Verification items for the finished model (mm, model axes). Face numbers are marked on the shaded views. Coordinates: 2 decimals unless noted, no trailing zeros. Order: outer loops, then holes, each group sorted by start corner. A loop starts at its lowest first (then second) coordinate and runs counter-clockwise, first axis right, second up. Notation, with made-up numbers: M -14.75,60.5 L 37.25,60.5 A26 ccw 37.25,79.5 Z; hole C 48.5,17 d5. An arc over 180 degrees is marked long. Return JSON: item names as keys, results as strings. Group by question number.
1. Material ranges on line 1 along Z through (x, y) = (3, 14.75); line 2 along Z through (x, y) = (3.75, 12.5); line 3 along X through (y, z) = (6, -2), recorded low to high.
2. Gauge pin test, flat ends, axial feed: pin 1 (2 mm diameter, centred on x = 3.5, z = -0.5, fed in from -Y); pin 2 (1.8 mm diameter, centred on x = 3.5, z = 2, fed in from +Y). Record the tip position at first contact, or that the pin passes through.
3. Section check D-D, the plane z = -1.25. Record the cut outline in (x, y).
4. Section check A-A, the plane x = 3.5. Record the cut outline in (y, z), plus the area to 3 significant figures.
5. Section check C-C, the plane z = -2.75. Record the cut outline in (x, y), plus the area to 3 significant figures.
6. Section check B-B, the plane y = 9. Record the cut outline in (x, z).
7. Mould release check, pull along X, two halves, no side actions. Record for the marked faces 1, 2 and 3: +X half, -X half, draft (parallel to the pull), parting line (faces both ways), or undercut.
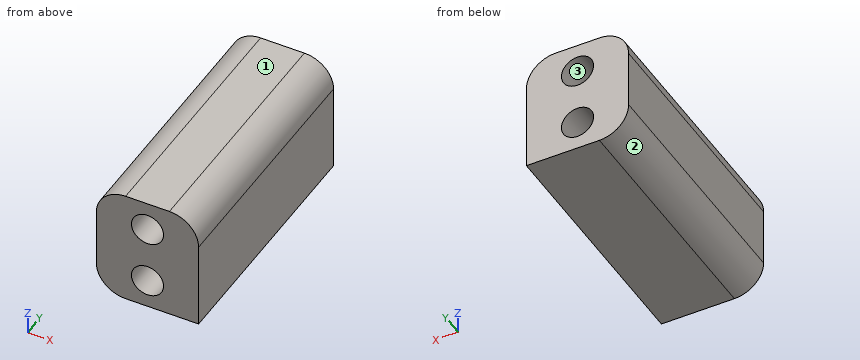
```python
from build123d import *

# Parameters (mm, degrees)
SKETCH_1_W      = 7
SKETCH_1_H      = 8
SKETCH_1_R      = 1.1
EXTRUDE_1_DEPTH = 17
FILLET_1_R      = 2


with BuildPart() as part:
    # 草图1 → 凸台-拉伸1 (new body)
    with BuildSketch(Plane(origin=(0, 0, 0), x_dir=(1, 0, 0), z_dir=(0, 1, 0))):
        with Locations((3.5, 0)):
            Rectangle(SKETCH_1_W, SKETCH_1_H)
        with Locations(Location((3.5, -2, 0), (0, 0, 270))):
            Circle(SKETCH_1_R, mode=Mode.SUBTRACT)
        with Locations(Location((3.5, 2, 0), (0, 0, 270))):
            Circle(SKETCH_1_R, mode=Mode.SUBTRACT)
    extrude(amount=EXTRUDE_1_DEPTH)

    # 圆角1
    fillet_1_edges = [part.edges().sort_by_distance(p)[0] for p in [
        (7, 8.5, 4),
        (0, 8.5, 4),
        (0, 8.5, -4),
    ]]
    fillet(fillet_1_edges, radius=FILLET_1_R)


solid = part.part
```
Answers follow:
{
 "1": {"line 1": "-4 to -2.98, -1.02 to 1.02, 2.98 to 4", "line 2": "-4 to -3.07, -0.93 to 0.93, 3.07 to 4", "line 3": "0 to 2.4, 4.6 to 7"},
 "2": {"pin 1": "y = 0", "pin 2": "through"},
 "3": {"outline": "M 0,0 L 2.7,0 L 2.7,17 L 0,17 Z; M 4.3,0 L 7,0 L 7,17 L 4.3,17 Z"},
 "4": {"outline": "M 0,-4 L 17,-4 L 17,-3.1 L 0,-3.1 Z; M 0,-0.9 L 17,-0.9 L 17,0.9 L 0,0.9 Z; M 0,3.1 L 17,3.1 L 17,4 L 0,4 Z", "area": "61.2 mm^2"},
 "5": {"outline": "M 0.15,0 L 2.7,0 L 2.7,17 L 0.15,17 Z; M 4.3,0 L 7,0 L 7,17 L 4.3,17 Z", "area": "89.2 mm^2"},
 "6": {"outline": "M 0,-2 A2 ccw 2,-4 L 7,-4 L 7,2 A2 ccw 5,4 L 2,4 A2 ccw 0,2 Z; hole C 3.5,-2 d2.2; hole C 3.5,2 d2.2"},
 "7": {"face 1": "draft", "face 2": "-X half", "face 3": "undercut"}
}
